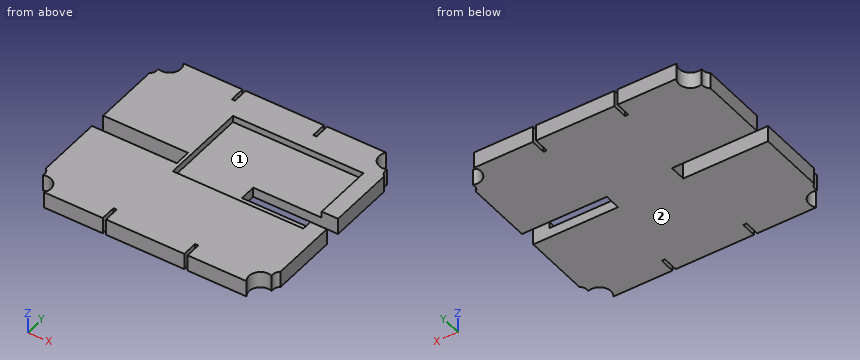
Autodesk Inventor part; units mm, degrees
ref_plane "YZ Plane" through (0, 0, 0) normal (1, 0, 0) x (0, 1, 0)
ref_plane "XZ Plane" through (0, 0, 0) normal (0, 1, 0) x (-1, 0, 0)
ref_plane "XY Plane" through (0, 0, 0) normal (0, 0, 1) x (1, 0, 0)
sketch "Эскиз1" plane through (0, 0, 0) normal (0, 0, 1) x (1, 0, 0)
  line L0 (174.3111, 41.624) -> (226.3111, 41.624)
  line L1 (134.3111, 31.624) -> (82.3111, 31.624)
  line L2 (174.3111, 41.624) -> (174.3111, 31.624)
  line L3 (149.3111, 46.624) -> (159.3111, 46.624)
  line L4 (149.3111, 46.624) -> (149.3111, 86.624)
  line L5 (149.3111, 86.624) -> (159.3111, 86.624)
  line L6 (159.3111, 86.624) -> (159.3111, 46.624)
  line L7 (134.3111, 31.624) -> (134.3111, 41.624)
  line L8 (226.3111, 31.624) -> (174.3111, 31.624)
  line L9 (82.3111, 41.624) -> (134.3111, 41.624)
  line L10 (226.3111, 41.624) -> (226.3111, 82.624)
  arc A0 (216.499, 98.624) -> (224.45, 87.7942) centre (222.0611, 94.374) ccw
  line L11 (216.499, 98.624) -> (180.3111, 98.624)
  line L12 (180.3111, 98.624) -> (180.3111, 89.124)
  line L13 (180.3111, 89.124) -> (178.3111, 89.124)
  line L14 (178.3111, 89.124) -> (178.3111, 98.624)
  line L15 (178.3111, 98.624) -> (130.3111, 98.624)
  line L16 (130.3111, 98.624) -> (130.3111, 89.124)
  line L17 (130.3111, 89.124) -> (128.3111, 89.124)
  line L18 (128.3111, 89.124) -> (128.3111, 98.624)
  line L19 (128.3111, 98.624) -> (92.1233, 98.624)
  arc A1 (84.1722, 87.7942) -> (92.1233, 98.624) centre (86.5611, 94.374) ccw
  line L20 (82.3111, -9.376) -> (82.3111, 31.624)
  arc A2 (92.1233, -25.376) -> (84.1722, -14.5463) centre (86.5611, -21.126) ccw
  line L21 (128.3111, -25.376) -> (92.1233, -25.376)
  line L22 (128.3111, -25.376) -> (128.3111, -15.876)
  line L23 (128.3111, -15.876) -> (130.3111, -15.876)
  line L24 (130.3111, -15.876) -> (130.3111, -25.376)
  line L25 (178.3111, -25.376) -> (130.3111, -25.376)
  line L26 (178.3111, -25.376) -> (178.3111, -15.876)
  line L27 (178.3111, -15.876) -> (180.3111, -15.876)
  line L28 (180.3111, -15.876) -> (180.3111, -25.376)
  line L29 (216.499, -25.376) -> (180.3111, -25.376)
  arc A3 (224.45, -14.5463) -> (216.499, -25.376) centre (222.0611, -21.126) ccw
  line L30 (159.3111, 26.624) -> (149.3111, 26.624)
  line L31 (159.3111, 26.624) -> (159.3111, -13.376)
  line L32 (159.3111, -13.376) -> (149.3111, -13.376)
  line L33 (149.3111, -13.376) -> (149.3111, 26.624)
  arc A4 (224.45, 87.7942) -> (226.3111, 82.624) centre (229.3111, 86.624) ccw
  arc A5 (84.1722, -14.5463) -> (82.3111, -9.376) centre (79.3111, -13.376) ccw
  arc A6 (82.3111, 82.624) -> (84.1722, 87.7942) centre (79.3111, 86.624) ccw
  arc A7 (226.3111, -9.376) -> (224.45, -14.5463) centre (229.3111, -13.376) ccw
  line L34 (226.3111, -9.376) -> (226.3111, 31.624)
  line L35 (82.3111, 41.624) -> (82.3111, 82.624)
  point P0 (0, 0)
  point P1 (179.3111, -15.876)
  point P2 (129.3111, -15.876)
  point P3 (70.835, 120.6534)
  point P4 (129.3111, 89.124)
  point P5 (179.3111, 89.124)
  point P6 (242.2845, 49.4059)
  point P7 (79.3111, -13.376)
  point P8 (229.3111, -13.376)
extrude "Выдавливание1" add sketch "Эскиз1" along normal blind 10 contours L2 L8 L34 A7 A3 L29 L28 L27 L26 L25 L24 L23 L22 L21 A2 A5 L20 L1 L7 L9 L35 A6 A1 L19 L18 L17 L16 L15 L14 L13 L12 L11 A0 A4 L10 L0 | L4 L5 L6 L3 | L31 L32 L33 L30
sketch "Эскиз2" plane through (0, 0, 10) normal (0, 0, 1) x (1, 0, 0)
  line L0 (216.3111, 25.284) -> (136.3111, 25.284)
  line L1 (136.3111, 25.284) -> (136.3111, 78.624)
  line L2 (136.3111, 78.624) -> (216.3111, 78.624)
  line L3 (216.3111, 78.624) -> (216.3111, 25.284)
  line L4 (226.3111, 41.624) -> (226.3111, 82.624)
  line L5 (216.499, 98.624) -> (180.3111, 98.624)
  point P0 (0, 0)
  point P1 (231.3111, -8.7934)
  point P2 (231.3111, 82.0414)
  point P3 (226.3111, 82.624)
  dimension "d14" = 80
  dimension "d15" = 53.34
  dimension "d58" = 20
  dimension "d59" = 10
extrude "Выдавливание2" cut sketch "Эскиз2" against normal blind 4
properties part number "Каркас"
For this review, take the finished solid that the model builds, in its own axes (mm). Face numbers are marked on the shaded views. Coordinates: 2 decimals unless noted, no trailing zeros. Write each loop counter-clockwise with the first axis right and the second up, starting at its lowest first coordinate (ties: lowest second). Pieces come first, ordered by that corner, then holes. Notation, with made-up numbers: (39, 56) - (51, 56) arc R30 cw to (51, 90) - close; hole circle Ø6 at (-39.5, 6). An arc over 180 degrees is marked (long way). Put each result on its own line as item: value.
1. Add section B-B, the plane y = 43.5. Give the boundary of the cut face in (x, z).
Values found:
outline: (82.31, 0) - (226.31, 0) - (226.31, 10) - (216.31, 10) - (216.31, 6) - (136.31, 6) - (136.31, 10) - (82.31, 10) - close
2. Add section A-A, the plane x = 201.5. Give the boundary of the cut face in (y, z), then the cut area to 3 significant figures.
Values found:
outline: (-25.38, 0) - (31.62, 0) - (31.62, 6) - (25.28, 6) - (25.28, 10) - (-25.38, 10) - close; (41.62, 0) - (98.62, 0) - (98.62, 10) - (78.62, 10) - (78.62, 6) - (41.62, 6) - close
area: 967 mm²
3. Add section D-D, the plane x = 148.5. Give the boundary of the cut face in (y, z).
Values found:
outline: (-25.38, 0) - (98.62, 0) - (98.62, 10) - (78.62, 10) - (78.62, 6) - (25.28, 6) - (25.28, 10) - (-25.38, 10) - close
4. Mouldability with a two-part tool opening along Y and no side actions: class the marked faces 1 and 2 as released by +Y, released by -Y, zero draft, split by the parting line, or undercut.
Values found:
face 1: undercut
face 2: zero draft
5. Add section C-C, the plane x = 122.5. Give the boundary of the cut face in (y, z), then the cut area to 3 significant figures.
Values found:
outline: (-25.38, 0) - (31.62, 0) - (31.62, 10) - (-25.38, 10) - close; (41.62, 0) - (98.62, 0) - (98.62, 10) - (41.62, 10) - close
area: 1,140 mm²
6. For pin 1 (3 mm diameter, centred on y = 94, z = 6.5, fed in from -X); pin 2 (3 mm diameter, centred on y = 34.5, z = 4.5, fed in from -X), all flat-tipped, find the tip position at first contact; note any pin that passes through.
Values found:
pin 1: x = 93.31
pin 2: x = 134.31
7. Wall thickness on probe 1 along Y at (x, z) = (201.5, 9); probe 2 along Y at (x, z) = (103.5, 4.5); probe 3 along X at (y, z) = (44.5, 7.25): over which ranges is each line inside the solid? List them lowest first.
Values found:
probe 1: -25.38 to 25.28, 78.62 to 98.62
probe 2: -25.38 to 31.62, 41.62 to 98.62
probe 3: 82.31 to 136.31, 216.31 to 226.31
